Build history of the part. All positions in model axes, mm. A direction names the side the tool comes from. Round coordinates to 2 decimals unless told otherwise and drop trailing zeros. Write each loop counter-clockwise with the first axis right and the second up, starting at its lowest first coordinate (ties: lowest second). Pieces come first, ordered by that corner, then holes.
from build123d import *

# Parameters (mm, degrees)
BOSS_EXTRUDE1_DEPTH = 1.6
SKETCH2_R           = 1.1
SKETCH2_R_2         = 0.822376014
BOSS_EXTRUDE2_DEPTH = 18
CUT_EXTRUDE1_START  = -2
SKETCH4_R           = 2.275
CUT_EXTRUDE1_DEPTH  = 18
SKETCH5_W           = 13.5
SKETCH5_H           = 16
CUT_EXTRUDE2_DEPTH  = 18
SKETCH6_W           = 44.533379649
SKETCH6_H           = 1.6
BOSS_EXTRUDE3_DEPTH = 6


with BuildPart() as part:
    # Sketch1 → Boss-Extrude1 (new body)
    with BuildSketch(Plane.XY):
        Polygon((-38.4, 43.8), (-38.4, 40.4), (-21, 40.4), (-21, 43.8), (0, 43.8), (0, 0), (-21, 0), (-21, 3.4), (-38.4, 3.4), (-38.4, 0), (-59.4, 0), (-59.4, 43.8), align=None)
    extrude(amount=BOSS_EXTRUDE1_DEPTH)

    # Sketch2 → Boss-Extrude2 (add)
    with BuildSketch(Plane.XY.offset(1.6)):
        Polygon((-59.4, 43.8), (-38.4, 43.8), (-38.4, 40.4), (-21, 40.4), (-21, 43.8), (0, 43.8), (0, 0), (-21, 0), (-21, 3.4), (-38.4, 3.4), (-38.4, 0), (-59.4, 0), align=None)
        with Locations((-57.8, 1.6)):
            Circle(SKETCH2_R, mode=Mode.SUBTRACT)
        with Locations((-57.8, 42.2)):
            Circle(SKETCH2_R, mode=Mode.SUBTRACT)
        with Locations((-1.6, 42.2)):
            Circle(SKETCH2_R, mode=Mode.SUBTRACT)
        with Locations((-1.6, 1.6)):
            Circle(SKETCH2_R_2, mode=Mode.SUBTRACT)
        with BuildLine():
            Line((-54.6, 42.2), (-40, 42.2))
            Line((-40, 42.2), (-40, 38.8))
            Line((-40, 38.8), (-19.4, 38.8))
            Line((-19.4, 38.8), (-19.4, 42.2))
            Line((-19.4, 42.2), (-4.8, 42.2))
            ThreePointArc((-4.8, 42.2), (-3.8627417, 39.9372583), (-1.6, 39))
            Line((-1.6, 39), (-1.6, 4.8))
            ThreePointArc((-1.6, 4.8), (-3.8627417, 3.8627417), (-4.8, 1.6))
            Line((-4.8, 1.6), (-19.4, 1.6))
            Line((-19.4, 1.6), (-19.4, 5))
            Line((-19.4, 5), (-40, 5))
            Line((-40, 5), (-40, 1.6))
            Line((-40, 1.6), (-54.6, 1.6))
            ThreePointArc((-54.6, 1.6), (-55.5372583, 3.8627417), (-57.8, 4.8))
            Line((-57.8, 4.8), (-57.8, 39))
            ThreePointArc((-57.8, 39), (-55.5372583, 39.9372583), (-54.6, 42.2))
        make_face(mode=Mode.SUBTRACT)
    extrude(amount=BOSS_EXTRUDE2_DEPTH)

    # Sketch4 → Cut-Extrude1 (cut)
    with BuildSketch(Plane.XY.offset(19.6).offset(CUT_EXTRUDE1_START)):
        with Locations((-57.8, 42.2)):
            Circle(SKETCH4_R)
        with Locations((-1.6, 42.2)):
            Circle(SKETCH4_R)
        with Locations((-57.8, 1.6)):
            Circle(SKETCH4_R)
        with Locations((-1.6, 1.6)):
            Circle(SKETCH4_R)
    extrude(amount=-CUT_EXTRUDE1_DEPTH, mode=Mode.SUBTRACT)

    # Sketch5 → Cut-Extrude2 (cut)
    with BuildSketch(Plane.ZY.offset(59.4)):
        with Locations((12.85, 21.9)):
            Rectangle(SKETCH5_W, SKETCH5_H)
    extrude(amount=-CUT_EXTRUDE2_DEPTH, mode=Mode.SUBTRACT)

    # Sketch6 → Boss-Extrude3 (add)
    with BuildSketch(Plane.XY.offset(1.6)):
        Polygon((-57.8, 33.4), (-3.8, 33.4), (-3.8, 10.4), (-3.8, 8.8), (-1.6, 8.8), (-1.6, 35), (-57.8, 35), align=None)
        with Locations((-35.533310176, 9.6)):
            Rectangle(SKETCH6_W, SKETCH6_H)
    extrude(amount=BOSS_EXTRUDE3_DEPTH)


solid = part.part
1) Slice it at A-A (x = -44). Write the cut outline in (y, z), plus the area to 3 significant figures.
Results:
outline: (0, 0) - (43.8, 0) - (43.8, 19.6) - (42.2, 19.6) - (42.2, 1.6) - (35, 1.6) - (35, 7.6) - (33.4, 7.6) - (33.4, 1.6) - (10.4, 1.6) - (10.4, 7.6) - (8.8, 7.6) - (8.8, 1.6) - (1.6, 1.6) - (1.6, 19.6) - (0, 19.6) - close
area: 147 mm2
2) Slice it at C-C (y = 7.5). Write the cut outline in (x, z).
Results:
outline: (-59.4, 0) - (0, 0) - (0, 19.6) - (-1.6, 19.6) - (-1.6, 1.6) - (-57.8, 1.6) - (-57.8, 19.6) - (-59.4, 19.6) - close
3) Which spindle directions (+Z, -Z, +X, -X, +Y, -Y) get a long thin tool onto all of the face, cutting with end or side? Do faces 5 (the flat face through (-11, 43.8, 10)), 6 (the flat face through (-3.8, 21, 5)). Say none if no direction does.
Results:
face 5: +Z, -Z, +X, -X, +Y
face 6: +Z
4) Slice it at B-B (y = 26). Write the cut outline in (x, z).
Results:
outline: (-59.4, 0) - (0, 0) - (0, 19.6) - (-1.6, 19.6) - (-1.6, 7.6) - (-3.8, 7.6) - (-3.8, 1.6) - (-57.8, 1.6) - (-57.8, 6.1) - (-59.4, 6.1) - close
5) Pin check, flat tips, straight feed: pin 1 Ø1.2 at (x, y) = (-57, 2.5) entering from -Z; pin 2 Ø6.5 at (x, z) = (-27, 6) entering from +Y; pin 3 Ø1.5 at (x, z) = (-36.5, 9) entering from -Y. Stop position of each tip, or through.
Results:
pin 1: stops at z = 17.6
pin 2: stops at y = 40.4
pin 3: stops at y = 3.4
6) Mould opens along Y. For faces 1 (the flat face through (-59.4, 22, 5)), 2 (the flat face through (-10, 0, 10)), 3 (the flat face through (-30, 40.4, 10)), 4 (the flat face through (-59, 22, 6.1)) say: released by +Y, released by -Y, zero draft, split by the parting line, or undercut.
Results:
face 1: zero draft
face 2: released by -Y
face 3: released by +Y
face 4: undercut
7) Slice it at D-D (z = 4.25). Count the separate pieces of the cut face and the enclosed holes in it, plus the area to 3 significant figures.
Results:
separate pieces: 1
enclosed holes: 2
area: 536 mm2
8) Wall check: L1, parallel to Y at x = -35.5, z = 8.75; L2, parallel to X at y = 41.5, z = 5.5; L3, parallel to Z at x = -6.5, y = 10. Give the ranges that are in metal, low to high.
Results:
L1: y = 3.4 to 5, 38.8 to 40.4
L2: x = -55.64 to -54.68, -40 to -38.4, -21 to -19.4, -4.72 to -3.76
L3: z = 0 to 1.6
